The listing builds one solid part. Answer for the finished solid, in the listing's coordinates (mm). A direction names the side the tool comes from. Give positions to 0.01 mm unless a question says otherwise; leave off trailing zeros. Order: outer loops, then holes, each group sorted by start corner. A loop starts at its lowest first (then second) coordinate and runs counter-clockwise, first axis right, second up. Notation, with made-up numbers: (-10.75, 17.25) - (4.25, 17.25) arc R19 cw to (4.25, 40.25) - close; hole circle Ø8 at (74.5, 75). An arc over 180 degrees is marked (long way). Answer as CSV lines item,"result". Start each with the question number.
1. Section A-A on x = -17 is taken. Give the vertices of the cut face in (y, z), and give its area (3 significant figures).
2. Flat-ended cylindrical pins translate along their axes: pin 1 (12 mm diameter, centred on y = -50.5, z = -13, fed in from -X); pin 2 (6 mm diameter, centred on x = 4.5, z = -30, fed in from -Y) (3 decimals); pin 3 (12 mm diameter, centred on x = 7, y = -37, fed in from +Z); pin 4 (18 mm diameter, centred on x = 0, y = 0, fed in from +Z). Find the tip coordinate at first contact, or state that the pin passes through.
3. Determine the mould class of faces 1 (the cylindrical face through (-14.985, 0.66, -0.56)), 2 (the flat face through (0, -17, -40)), 3 (the flat face through (0.14, -33.8, 19.48)) for opening direction Y: +Y half, -Y half, draft (parallel to the pull), parting line (faces both ways), or undercut.
4. Section D-D on z = 22 is taken. Give the vertices of the cut face in (x, y).
5. Which of the six approach directions +Z, -Z, +X, -X, +Y, -Y give full straight-line access (tool end or side, diameter ignored) to faces 4 (the flat face through (0, -51, 0)), 5 (the flat face through (-20, -66, -29)), 6 (the flat face through (20, -66, -29))?
6. Section C-C on y = -47.5 is taken. Give the vertices of the cut face in (x, z), and give its area (3 significant figures).
7. Consider line 1 along Z through (x, y) = (-2.75, -57); line 2 along Y through (x, z) = (12, -23); line 3 along Y through (x, z) = (-9, -12). Determine where each line is inside the solid, lowest interval first. Write a range as [from, to].
8. Section B-B on z = -10.5 is taken. Give the vertices of the cut face in (x, y), and give its area (3 significant figures).
from build123d import *

# Parameters (mm, degrees)
F0_R     = 25
F0_R_2   = 15
F1_DEPTH = 40
F2_R     = 12.5
F3_DEPTH = 10
F4_DEPTH = 20


with BuildPart() as f1:
    # F0 (on Top) → F1 (new body, symmetric)
    with BuildSketch(Plane.XY):
        Circle(F0_R)
        Circle(F0_R_2, mode=Mode.SUBTRACT)
    extrude(amount=F1_DEPTH, both=True)

    # F2 (on Right) → F3 (join, symmetric)
    with BuildSketch(Plane.YZ):
        with BuildLine():
            ThreePointArc((-57, -40), (-42.8578643763, -34.1421356237), (-37, -20))
            ThreePointArc((-37, -20), (-42.8578643763, -5.8578643763), (-57, 0))
            ThreePointArc((-57, 0), (-77, -20), (-57, -40))
        make_face()
        with Locations((-57, -20)):
            Circle(F2_R, mode=Mode.SUBTRACT)
        with BuildLine():
            ThreePointArc((-57, 0), (-42.8578643763, -5.8578643763), (-37, -20))
            ThreePointArc((-37, -20), (-42.8578643763, -34.1421356237), (-57, -40))
            Line((-57, -40), (-22, -40))
            Line((-22, -40), (-22, 0))
            Line((-22, 0), (-45, 0))
            Line((-45, 0), (-57, 0))
        make_face()
        Polygon((-22, 40), (-45, 0), (-22, 0), align=None)
    extrude(amount=F3_DEPTH, both=True)

    # F2 (on Right) → F4 (join, symmetric)
    with BuildSketch(Plane.YZ):
        with BuildLine():
            ThreePointArc((-57, -40), (-42.8578643763, -34.1421356237), (-37, -20))
            ThreePointArc((-37, -20), (-42.8578643763, -5.8578643763), (-57, 0))
            ThreePointArc((-57, 0), (-77, -20), (-57, -40))
        make_face()
        with Locations((-57, -20)):
            Circle(F2_R, mode=Mode.SUBTRACT)
    extrude(amount=F4_DEPTH, both=True)


solid = f1.part
Checks:
1,outline,"circle Ø40 at (-57, -20); (-18.33, -40) - (18.33, -40) - (18.33, 40) - (-18.33, 40) - close; hole circle Ø25 at (-57, -20)"
1,area,"3,700 mm²"
2,pin 1,"stops at x = -20"
2,pin 2,"stops at y = -75.735"
2,pin 3,"stops at z = 24.35"
2,pin 4,"passes through"
3,face 1,"undercut"
3,face 2,"draft"
3,face 3,"-Y half"
4,outline,"(-10, -32.35) - (10, -32.35) - (10, -22.91) arc R25 ccw (long way) to (-10, -22.91) - close; hole circle Ø30 at (0, 0)"
5,face 4,"+Z, +X, -X, -Y"
5,face 5,"+Z, -Z, -X, -Y"
5,face 6,"+Z, -Z, +X, -Y"
6,outline,"(-20, -37.6) - (-10, -37.6) - (-10, -40) - (10, -40) - (10, -37.6) - (20, -37.6) - (20, -28.12) - (-20, -28.12) - close; (-20, -11.88) - (20, -11.88) - (20, -2.4) - (10, -2.4) - (10, 0) - (-10, 0) - (-10, -2.4) - (-20, -2.4) - close"
6,area,"854 mm²"
7,line 1,"z = [-40, -32.5], [-7.5, 0]"
7,line 2,"y = [-76.77, -69.13], [-44.87, -37.23], [-21.93, -9], [9, 21.93]"
7,line 3,"y = [-75.33, -66.6], [-47.4, -12], [12, 23.32]"
8,outline,"(-20, -74.6) - (20, -74.6) - (20, -65.12) - (-20, -65.12) - close; (-20, -48.88) - (20, -48.88) - (20, -39.4) - (10, -39.4) - (10, -22.91) arc R25 ccw (long way) to (-10, -22.91) - (-10, -39.4) - (-20, -39.4) - close; hole circle Ø30 at (0, 0)"
8,area,"2,320 mm²"
